Read the model definition and answer for the solid it produces. Units are mm, in the model's axes. A direction names the side the tool comes from. Coordinates: 2 decimals unless noted, no trailing zeros. Write each loop counter-clockwise with the first axis right and the second up, starting at its lowest first coordinate (ties: lowest second). Pieces come first, ordered by that corner, then holes. Notation, with made-up numbers: (43, 81) -> (65, 81) arc R17 cw to (65, 102) -> close; hole circle Ø5 at (-3.75, -36.75). An arc over 180 degrees is marked (long way). Answer as a JSON object with one key per item and string values. Group by question number.
(1) Find section C-C (z = 20.5). Give the vertices of the cut face in (x, y).
(2) Which of the six approach directions +Z, -Z, +X, -X, +Y, -Y give full straight-line access (tool end or side, diameter ignored) to faces 1 (the face through (67, 18, 22)), 2 (the face through (-76, 20, 6)), 3 (the face through (-14, 3, 40)), 4 (the face through (89, 20, -25)), 5 (the face through (-67, 18, -22))?
(3) Find section D-D (z = -38.5). Give the vertices of the cut face in (x, y).
(4) Find section A-A (y = 9). Give the vertices of the cut face in (x, z).
(5) For a pull along Z with two mould halves and no side action, classify faces 6 (the face through (-14, 0, 41)), 7 (the face through (-89, 20, 25)), 8 (the face through (79, 20, -3)) as +Z half, -Z half, draft (parallel to the pull), parting line (faces both ways), or undercut.
(6) Flat-ended cylindrical pins translate along their axes: P1, Ø6.5, axis at x = 48, z = -39, coming from the +Y side; P2, Ø5, axis at y = 22.5, z = 21, coming from the +X side; P3, Ø0.9, axis at y = 1, z = -38.5, coming from the +X side. Find the tip coordinate at first contact, or state that the pin passes through.
(7) Find section B-B (x = 74). Give the vertices of the cut face in (y, z).
(8) Straight lines are drawn through the part: L1, parallel to Z at x = -58.5, y = 13; L2, parallel to X at y = 16.5, z = 20.5; L3, parallel to Z at x = -79.5, y = 16.5. For each, find the intervals that lie inside material, in ascending order.
from build123d import *

# Parameters (mm, degrees)
BOSS_EXTRUDE1_DEPTH = 3
BOSS_EXTRUDE2_DEPTH = 22
SKETCH3_W           = 88
SKETCH3_H           = 19.19179848
CUT_EXTRUDE1_DEPTH  = 208
SKETCH5_W           = 153
SKETCH5_H           = 8
BOSS_EXTRUDE3_DEPTH = 3


with BuildPart() as part:
    # Sketch1 → Boss-Extrude1 (new body)
    with BuildSketch(Plane(origin=(0, 0, 0), x_dir=(1, 0, 0), z_dir=(0, 1, 0))):
        Polygon((-92, -3), (-92, -47), (-67, -47), (67, -47), (67, 3), (92, 3), (92, 47), (-67, 47), (-67, -3), align=None)
    extrude(amount=BOSS_EXTRUDE1_DEPTH)

    # Sketch2 → Boss-Extrude2 (add)
    with BuildSketch(Plane(origin=(0, 3, 0), x_dir=(1, 0, 0), z_dir=(0, 1, 0))):
        Polygon((92, 3), (92, 47), (-67, 47), (-67, -3), (-92, -3), (-92, -47), (67, -47), (67, 3), align=None)
        Polygon((-64, 44), (-64, -6), (-89, -6), (-89, -44), (64, -44), (64, 6), (89, 6), (89, 44), align=None, mode=Mode.SUBTRACT)
    extrude(amount=BOSS_EXTRUDE2_DEPTH)

    # Sketch3 → Cut-Extrude1 (cut)
    with BuildSketch(Plane(origin=(92, 0, 0), x_dir=(0, 0, -1), z_dir=(1, 0, 0))):
        with Locations((0, 5.40410076)):
            Rectangle(SKETCH3_W, SKETCH3_H)
    extrude(amount=-CUT_EXTRUDE1_DEPTH, mode=Mode.SUBTRACT)

    # Sketch5 → Boss-Extrude3 (add)
    with BuildSketch(Plane.XZ):
        with Locations((-12.5, 40)):
            Rectangle(SKETCH5_W, SKETCH5_H)
        with Locations((12.5, -40)):
            Rectangle(SKETCH5_W, SKETCH5_H)
    extrude(amount=-BOSS_EXTRUDE3_DEPTH)


solid = part.part
Results below:
{
 "1": {"outline": "(-92, 15) -> (-89, 15) -> (-89, 25) -> (-92, 25) -> close; (64, 15) -> (67, 15) -> (67, 25) -> (64, 25) -> close"},
 "2": {"face 1": "+Z, +X, +Y, -Y", "face 2": "+Y, -Y", "face 3": "+X, -X, +Y", "face 4": "+Y", "face 5": "-Z, -X, +Y, -Y"},
 "3": {"outline": "(-67, 15) -> (-64, 15) -> (-64, 25) -> (-67, 25) -> close; (-64, 0) -> (89, 0) -> (89, 3) -> (-64, 3) -> close; (89, 15) -> (92, 15) -> (92, 25) -> (89, 25) -> close"},
 "4": {"outline": "(-92, 44) -> (67, 44) -> (67, 47) -> (-92, 47) -> close; (-67, -47) -> (92, -47) -> (92, -44) -> (-67, -44) -> close"},
 "5": {"face 6": "draft", "face 7": "undercut", "face 8": "+Z half"},
 "6": {"P1": "stops at y = 3", "P2": "stops at x = 67", "P3": "stops at x = 89"},
 "7": {"outline": "(0, -47) -> (25, -47) -> (25, -44) -> (3, -44) -> (3, -36) -> (0, -36) -> close; (15, -6) -> (25, -6) -> (25, -3) -> (15, -3) -> close"},
 "8": {"L1": "z = -47 to -44, 44 to 47", "L2": "x = -92 to -89, 64 to 67", "L3": "z = 3 to 6, 44 to 47"}
}
